Source: CAD feature listing. Evaluate the final solid. Frame: model axes, mm. A direction names the side the tool comes from. Give positions to 0.01 mm unless a question says otherwise; leave off trailing zeros. Order: outer loops, then holes, each group sorted by start corner. A loop starts at its lowest first (then second) coordinate and runs counter-clockwise, first axis right, second up.
```python
from build123d import *

# Parameters (mm, degrees)
SKETCH_1_W          = 11
SKETCH_1_H          = 6
SKETCH_1_W_2        = 13
SKETCH_1_H_2        = 8
EXTRUDE_1_DEPTH     = 1.5
CUT_EXTRUDE_1_DEPTH = 1.5
FILLET_1_R          = 2
FILLET_2_R          = 1
SKETCH_3_R          = 0.8
CUT_EXTRUDE_2_DEPTH = 10
EXTRUDE_2_DEPTH     = 1
SKETCH_5_R          = 1.55
CUT_EXTRUDE_3_DEPTH = 10


with BuildPart() as part:
    # 草图1 → 凸台-拉伸1 (new body)
    with BuildSketch(Plane(origin=(0, 0, 0), x_dir=(1, 0, 0), z_dir=(0, 1, 0))):
        with Locations((-12, 0)):
            Rectangle(SKETCH_1_W, SKETCH_1_H)
        with Locations((0, -7)):
            Rectangle(SKETCH_1_W_2, SKETCH_1_H_2)
        Rectangle(SKETCH_1_W_2, SKETCH_1_H)
        with Locations((0, 7)):
            Rectangle(SKETCH_1_W_2, SKETCH_1_H_2)
        with Locations((12, 0)):
            Rectangle(SKETCH_1_W, SKETCH_1_H)
    extrude(amount=EXTRUDE_1_DEPTH)

    # 草图2 → 切除-拉伸1 (cut)
    with BuildSketch(Plane(origin=(0, 1.5, 0), x_dir=(1, 0, 0), z_dir=(0, 1, 0))):
        with BuildLine():
            Line((-5, -10), (5, -10))
            Line((5, -10), (5, -1.113552873))
            ThreePointArc((5, -1.113552873), (1.9, 0), (5, 1.113552873))
            Line((5, 1.113552873), (5, 10))
            Line((5, 10), (-5, 10))
            Line((-5, 10), (-5, 1.113552873))
            ThreePointArc((-5, 1.113552873), (-1.9, 0), (-5, -1.113552873))
            Line((-5, -1.113552873), (-5, -10))
        make_face()
    extrude(amount=-CUT_EXTRUDE_1_DEPTH, mode=Mode.SUBTRACT)

    # 圆角1
    fillet_1_edges = [part.edges().sort_by_distance(p)[0] for p in [
        (5, 0.75, -1.113552873),
        (5, 0.75, 1.113552873),
        (-5, 0.75, 1.113552873),
        (-5, 0.75, -1.113552873),
    ]]
    fillet(fillet_1_edges, radius=FILLET_1_R)

    # 圆角2
    fillet_2_edges = [part.edges().sort_by_distance(p)[0] for p in [
        (-6.5, 0.75, -3),
        (-6.5, 0.75, -11),
        (6.5, 0.75, -11),
        (6.5, 0.75, -3),
        (17.5, 0.75, -3),
        (17.5, 0.75, 3),
        (6.5, 0.75, 3),
        (6.5, 0.75, 11),
        (-6.5, 0.75, 11),
        (-6.5, 0.75, 3),
        (-17.5, 0.75, 3),
        (-17.5, 0.75, -3),
        (5, 0.75, -10),
        (5, 0.75, 10),
        (-5, 0.75, 10),
        (-5, 0.75, -10),
    ]]
    fillet(fillet_2_edges, radius=FILLET_2_R)

    # 草图3 → 切除-拉伸2 (cut)
    with BuildSketch(Plane(origin=(0, 1.5, 0), x_dir=(1, 0, 0), z_dir=(0, 1, 0))):
        with Locations(Location((-3.65, 0, 0), (0, 0, 270))):
            Circle(SKETCH_3_R)
        with Locations(Location((3.65, 0, 0), (0, 0, 270))):
            Circle(SKETCH_3_R)
    extrude(amount=-CUT_EXTRUDE_2_DEPTH, mode=Mode.SUBTRACT)

    # 草图4 → 凸台-拉伸2 (add)
    with BuildSketch(Plane(origin=(0, 1.5, 0), x_dir=(1, 0, 0), z_dir=(0, 1, 0))):
        with BuildLine():
            Line((-6.5, -4), (-6.5, 4))
            Line((-6.5, 4), (-6.5, 10))
            ThreePointArc((-6.5, 10), (-6.207106781, 10.707106781), (-5.5, 11))
            Line((-5.5, 11), (5.5, 11))
            ThreePointArc((5.5, 11), (6.207106781, 10.707106781), (6.5, 10))
            Line((6.5, 10), (6.5, 4))
            Line((6.5, 4), (6.5, -4))
            Line((6.5, -4), (6.5, -10))
            ThreePointArc((6.5, -10), (6.207106781, -10.707106781), (5.5, -11))
            Line((5.5, -11), (-5.5, -11))
            ThreePointArc((-5.5, -11), (-6.207106781, -10.707106781), (-6.5, -10))
            Line((-6.5, -10), (-6.5, -4))
        make_face()
        with BuildLine():
            Line((5, -3.693237063), (5, 9))
            ThreePointArc((5, 9), (4.707106781, 9.707106781), (4, 10))
            Line((4, 10), (-4, 10))
            ThreePointArc((-4, 10), (-4.707106781, 9.707106781), (-5, 9))
            Line((-5, 9), (-5, -3.693237063))
            Line((-5, -3.693237063), (-5, -9))
            ThreePointArc((-5, -9), (-4.707106781, -9.707106781), (-4, -10))
            Line((-4, -10), (4, -10))
            ThreePointArc((4, -10), (4.707106781, -9.707106781), (5, -9))
            Line((5, -9), (5, -3.693237063))
        make_face(mode=Mode.SUBTRACT)
    extrude(amount=EXTRUDE_2_DEPTH)

    # 草图5 → 切除-拉伸3 (cut)
    with BuildSketch(Plane.XZ):
        with Locations(Location((-13, 0, 0), (0, 0, 270))):
            Circle(SKETCH_5_R)
        with Locations(Location((13, 0, 0), (0, 0, 90))):
            Circle(SKETCH_5_R)
    extrude(amount=-CUT_EXTRUDE_3_DEPTH, mode=Mode.SUBTRACT)


solid = part.part
```
1) Section query D-D, the plane z = 0. Count the separate pieces of the cut face and the enclosed holes in it, and give its area (3 significant figures).
Report:
separate pieces: 6
enclosed holes: 0
area: 35.7 mm2
2) Reachability of faces 4 (the flat face through (-11, 1.5, 0)), 5 (the flat face through (0, 1, -10)), 6 (the flat face through (12, 1, -3)) from +Z, -Z, +X, -X, +Y, -Y: full face, straight path, thin tool, end or side. Return the list, or none.
Report:
face 4: +Z, -Z, -X, +Y
face 5: +Y, -Y
face 6: -Z, +X, +Y, -Y
3) Section query A-A, the plane x = 13. Return the cut outline in (y, z).
Report:
outline: (0, -3) - (1.5, -3) - (1.5, -1.55) - (0, -1.55) - close; (0, 1.55) - (1.5, 1.55) - (1.5, 3) - (0, 3) - close
4) Material intervals for L1, parallel to Z at x = 13, y = 0.85; L2, parallel to Z at x = -0.5, y = 1.2; L3, parallel to Z at x = -3, y = 0.75, sorted ascending.
Report:
L1: z = -3 to -1.55, 1.55 to 3
L2: z = -11 to -10, 10 to 11
L3: z = -11 to -10, -1.62 to -0.47, 0.47 to 1.62, 10 to 11
5) Section query C-C, the plane z = -8.25. Return the cut outline in (x, y), and give its area (3 significant figures).
Report:
outline: (-6.5, 0) - (-5, 0) - (-5, 2.5) - (-6.5, 2.5) - close; (5, 0) - (6.5, 0) - (6.5, 2.5) - (5, 2.5) - close
area: 7.50 mm2
6) Draft query along X for faces 1 (the flat face through (11, 1.5, 0)), 2 (the cylindrical face through (-17.215, 0.76, 2.699)), 3 (the cylindrical face through (-4.54, 0.74, -2.42)). Return one class per face: +X half, -X half, draft (parallel to the pull), parting line (faces both ways), or undercut.
Report:
face 1: draft
face 2: -X half
face 3: undercut
7) Section query B-B, the plane y = 2.05. Return the cut outline in (x, z), and give its area (3 significant figures).
Report:
outline: (-6.5, -10) arc R1 ccw to (-5.5, -11) - (5.5, -11) arc R1 ccw to (6.5, -10) - (6.5, 10) arc R1 ccw to (5.5, 11) - (-5.5, 11) arc R1 ccw to (-6.5, 10) - close; hole (-5, -9) arc R1 ccw to (-4, -10) - (4, -10) arc R1 ccw to (5, -9) - (5, 9) arc R1 ccw to (4, 10) - (-4, 10) arc R1 ccw to (-5, 9) - close
area: 86.0 mm2
8) Pin query (flat end, axial travel): pin 1 (1.2 mm diameter, centred on x = 12, y = 1, fed in from -Z); pin 2 (5 mm diameter, centred on x = 0, z = -3.5, fed in from -Y); pin 3 (0.9 mm diameter, centred on x = 4, z = 1.5, fed in from +Y); pin 4 (0.8 mm diameter, centred on x = 10, y = 1, fed in from +Z). Return the tip coordinate at first contact, or that it passes through.
Report:
pin 1: stops at z = -3
pin 2: passes through
pin 3: stops at y = 1.5
pin 4: stops at z = 3
